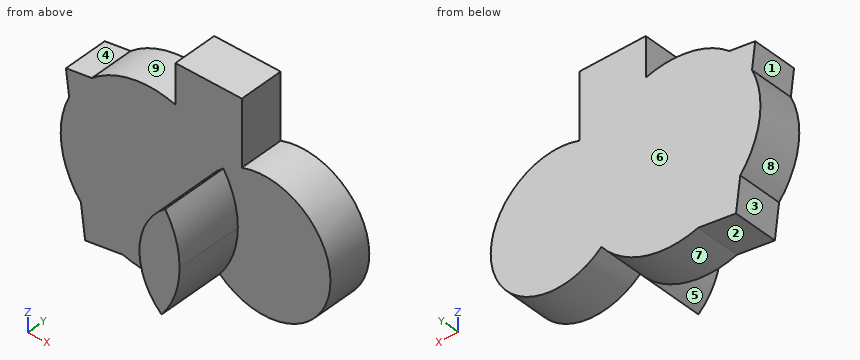
```python
from build123d import *

# Parameters (mm, degrees)
F1_DEPTH = 63.5
F2_DEPTH = 25.4


with BuildPart() as f1:
    # F0 (on Front) → F1 (new body)
    with BuildSketch(Plane.XZ):
        with BuildLine():
            ThreePointArc((-23.3141587542, 30.1340339415), (-38.0755183423, 1.3656145011), (-25.4130490193, -28.3863865178))
            ThreePointArc((-25.4130490193, -28.3863865178), (-17.7108136139, -13.8618974825), (-15.0505260944, 2.3617914412))
            ThreePointArc((-15.0505260944, 2.3617914412), (-17.1602423569, 16.849588705), (-23.3141587542, 30.1340339415))
        make_face()
    extrude(amount=F1_DEPTH)

    # F0 (on Front) → F2 (join)
    with BuildSketch(Plane.XZ):
        with BuildLine():
            ThreePointArc((-25.4130490193, -28.3863865178), (15.5462669532, -34.7839558391), (38.1, 0))
            ThreePointArc((38.1, 0), (21.9754793771, 31.1237579053), (-12.7497798503, 35.903385826))
            ThreePointArc((-12.7497798503, 35.903385826), (-18.2612505653, 33.4385515205), (-23.3141587542, 30.1340339415))
            ThreePointArc((-23.3141587542, 30.1340339415), (-17.1602423569, 16.849588705), (-15.0505260944, 2.3617914412))
            ThreePointArc((-15.0505260944, 2.3617914412), (-17.7108136139, -13.8618974825), (-25.4130490193, -28.3863865178))
        make_face()
        with BuildLine():
            ThreePointArc((-23.3141587542, 30.1340339415), (-18.2612505653, 33.4385515205), (-12.7497798503, 35.903385826))
            Line((-12.7497798503, 35.903385826), (-12.7497798503, 73.5738801328))
            Line((-12.7497798503, 73.5738801328), (-50.8497798503, 73.5738801328))
            Line((-50.8497798503, 73.5738801328), (-50.8497798503, 50.8964966749))
            ThreePointArc((-50.8497798503, 50.8964966749), (-35.2662192591, 42.9233517589), (-23.3141587542, 30.1340339415))
        make_face()
        with BuildLine():
            ThreePointArc((-80.903409919, -46.156768807), (-50.357269003, -46.0179458948), (-25.4130490193, -28.3863865178))
            ThreePointArc((-25.4130490193, -28.3863865178), (-38.0755183423, 1.3656145011), (-23.3141587542, 30.1340339415))
            ThreePointArc((-23.3141587542, 30.1340339415), (-35.2662192591, 42.9233517589), (-50.8497798503, 50.8964966749))
            Line((-50.8497798503, 50.8964966749), (-50.8497798503, 48.1738801328))
            Line((-50.8497798503, 48.1738801328), (-39.8230887478, -40.0396227074))
            Line((-39.8230887478, -40.0396227074), (-80.903409919, -46.156768807))
        make_face()
        with BuildLine():
            ThreePointArc((-23.3141587542, 30.1340339415), (-38.0755183423, 1.3656145011), (-25.4130490193, -28.3863865178))
            ThreePointArc((-25.4130490193, -28.3863865178), (-17.7108136139, -13.8618974825), (-15.0505260944, 2.3617914412))
            ThreePointArc((-15.0505260944, 2.3617914412), (-17.1602423569, 16.849588705), (-23.3141587542, 30.1340339415))
        make_face()
        with BuildLine():
            ThreePointArc((-105.0628087076, -29.9342902447), (-94.1695881341, -39.8124984188), (-80.903409919, -46.156768807))
            Line((-80.903409919, -46.156768807), (-39.8230887478, -40.0396227074))
            Line((-39.8230887478, -40.0396227074), (-50.8497798503, 48.1738801328))
            Line((-50.8497798503, 48.1738801328), (-98.7899056875, 41.0352613143))
            ThreePointArc((-98.7899056875, 41.0352613143), (-106.2058423832, 33.2177219447), (-111.8060832271, 24.0118900236))
            Line((-111.8060832271, 24.0118900236), (-105.0628087076, -29.9342902447))
        make_face()
        with BuildLine():
            Line((-102.6305822497, -49.3920961777), (-80.903409919, -46.156768807))
            ThreePointArc((-80.903409919, -46.156768807), (-94.1695881341, -39.8124984188), (-105.0628087076, -29.9342902447))
            Line((-105.0628087076, -29.9342902447), (-102.6305822497, -49.3920961777))
        make_face()
        with BuildLine():
            Line((-50.8497798503, 48.1738801328), (-50.8497798503, 50.8964966749))
            ThreePointArc((-50.8497798503, 50.8964966749), (-76.0857413983, 52.120010538), (-98.7899056875, 41.0352613143))
            Line((-98.7899056875, 41.0352613143), (-50.8497798503, 48.1738801328))
        make_face()
        with BuildLine():
            ThreePointArc((-111.8060832271, 24.0118900236), (-116.2582420031, -3.939174903), (-105.0628087076, -29.9342902447))
            Line((-105.0628087076, -29.9342902447), (-111.8060832271, 24.0118900236))
        make_face()
        with BuildLine():
            ThreePointArc((-111.8060832271, 24.0118900236), (-106.2058423832, 33.2177219447), (-98.7899056875, 41.0352613143))
            Line((-98.7899056875, 41.0352613143), (-113.6572733521, 38.8214066625))
            Line((-113.6572733521, 38.8214066625), (-111.8060832271, 24.0118900236))
        make_face()
    extrude(amount=F2_DEPTH)


solid = f1.part
```
Here's how the part is built. I have some questions about the finished solid (model axes, mm). Face numbers are marked on the shaded views. A direction names the side the tool comes from. Round coordinates to 2 decimals unless told otherwise and drop trailing zeros. Write each loop counter-clockwise with the first axis right and the second up, starting at its lowest first coordinate (ties: lowest second). Pieces come first, ordered by that corner, then holes.
Q1. Which directions (+Z, -Z, +X, -X, +Y, -Y) give clear straight access to the entire face, cutting with the end or side of a thin tool? Please do the marked faces 1, 2, 3, 4 and 5.
Q2. If we section it at A-A on y = -20: Write out the boundary of the cut face in (x, z).
Q3. If we section it at C-C on x = 0: Write out the boundary of the cut face in (y, z).
Q4. If we section it at D-D on y = -31: Write out the boundary of the cut face in (x, z).
Q5. Will these pins go through, and if not, where does the flat tip stop? P1, Ø3, axis at y = -17.5, z = -8, coming from the +X side; P2, Ø10, axis at x = 7.5, y = -29, coming from the +Z side; P3, Ø3, axis at x = -22.5, z = -4.5, coming from the +Y side; P4, Ø11.5, axis at y = -11, z = 67, coming from the -X side.
Q6. Please list where these lines run through material, in increasing order: probe 1 along Y at (x, z) = (8, -17.5); probe 2 along Z at (x, y) = (-32, -4); probe 3 along X at (y, z) = (-52.5, 4).
Q7. If we mould it in two halves opening along X, with no side actions, what happens to the marked faces 6, 7, 8 and 9? For each: +X half, -X half, draft (parallel to the pull), parting line (faces both ways), or undercut.
Q8. If we section it at B-B on z = -9: Write out the boundary of the cut face in (x, y).
Answer below:
1. face 1: -X, +Y, -Y
1. face 2: -Z, +Y, -Y
1. face 3: -Z, -X, +Y, -Y
1. face 4: +Z, -X, +Y, -Y
1. face 5: -X, -Y
2. outline: (-113.66, 38.82) - (-111.81, 24.01) arc R50.8 ccw to (-105.06, -29.93) - (-102.63, -49.39) - (-80.9, -46.16) arc R50.8 ccw to (-25.41, -28.39) arc R38.1 ccw (long way) to (-12.75, 35.9) - (-12.75, 73.57) - (-50.85, 73.57) - (-50.85, 50.9) arc R50.8 ccw to (-98.79, 41.04) - close
3. outline: (-25.4, -38.1) - (0, -38.1) - (0, 38.1) - (-25.4, 38.1) - close
4. outline: (-25.41, -28.39) arc R50.8 ccw to (-23.31, 30.13) arc R38.1 ccw to start
5. P1: stops at x = 37.54
5. P2: stops at z = 37.89
5. P3: stops at y = 0
5. P4: stops at x = -50.85
6. probe 1: y = -25.4 to 0
6. probe 2: z = -35.52 to 73.57
6. probe 3: x = -37.89 to -15.08
7. face 6: draft
7. face 7: undercut
7. face 8: -X half
7. face 9: undercut
8. outline: (-115.36, -25.4) - (-37.02, -25.4) - (-37.02, -63.5) - (-16.34, -63.5) - (-16.34, -25.4) - (37.02, -25.4) - (37.02, 0) - (-115.36, 0) - close
